Print and shaded views of the part. All mm, measured from the part's lowest x, y and z. A direction names the side the tool comes from. Round coordinates to 2 decimals unless told otherwise and drop trailing zeros. Loops run counter-clockwise (first coordinate to the right, second up) from the corner with the lowest first, then second, coordinate; pieces in that order, holes last. Notation, with made-up numbers: (-24.75, 26) - (-16.75, 26) arc R21 cw to (-16.75, 47) - close; hole circle Ø5 at (83.5, 71). An arc over 180 degrees is marked (long way). Use one line per item in the form item = value.
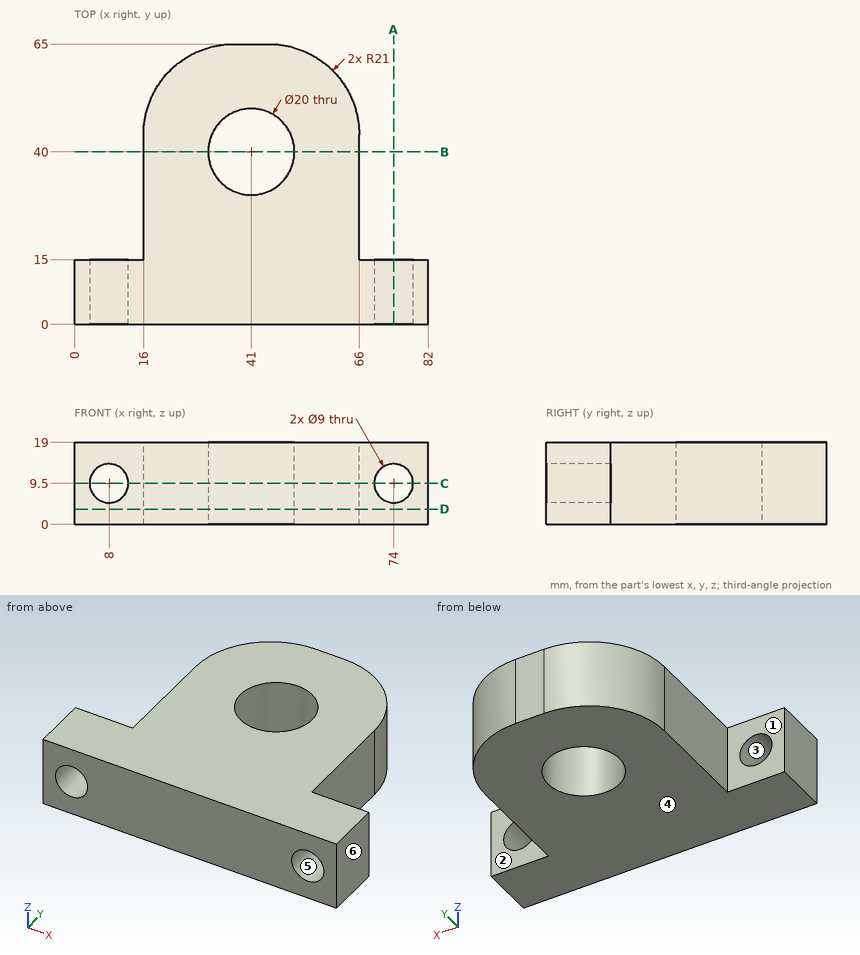
1) Flat gauge pins, fed straight in: pin 1 (1.5 mm diameter, centred on x = 10.5, z = 3.5, fed in from +Y); pin 2 (1 mm diameter, centred on y = 21, z = 7, fed in from +X); pin 3 (9.5 mm diameter, centred on y = 25, z = 10, fed in from -X). Where does each tip first touch, or does it go through?
Report:
pin_1 = 15
pin_2 = 66
pin_3 = 16
2) Slice it at C-C (z = 9.5). Write the cut outline in (x, y).
Report:
outline = (0, 0) - (3.5, 0) - (3.5, 15) - (0, 15) - close; (12.5, 0) - (69.5, 0) - (69.5, 15) - (66, 15) - (66, 44) arc R21 ccw to (45, 65) - (37, 65) arc R21 ccw to (16, 44) - (16, 15) - (12.5, 15) - close; (78.5, 0) - (82, 0) - (82, 15) - (78.5, 15) - close; hole circle Ø20 at (41, 40)
3) Tool access for the marked faces 1, 2 and 3: list every direction of +Z, -Z, +X, -X, +Y, -Y with a clear straight run to the whole face (end or side of a thin tool).
Report:
face_1 = +Z, -Z, -X, +Y
face_2 = +Z, -Z, +X, +Y
face_3 = +Y, -Y
4) Slice it at D-D (z = 3.5). Write the cut outline in (x, y).
Report:
outline = (0, 0) - (82, 0) - (82, 15) - (66, 15) - (66, 44) arc R21 ccw to (45, 65) - (37, 65) arc R21 ccw to (16, 44) - (16, 15) - (0, 15) - close; hole circle Ø20 at (41, 40)
5) Drill centre lines: probe 1 along Z at (x, y) = (74, 7); probe 2 along Y at (x, z) = (41, 7.5); probe 3 along Y at (x, z) = (71.5, 2.25). Where is each one in solid material? Low to high.
Report:
probe_1 = 0 to 5, 14 to 19
probe_2 = 0 to 30, 50 to 65
probe_3 = 0 to 15
6) Slice it at A-A (x = 74). Write the cut outline in (y, z).
Report:
outline = (0, 0) - (15, 0) - (15, 5) - (0, 5) - close; (0, 14) - (15, 14) - (15, 19) - (0, 19) - close
7) Two-plate mould, pull along Z, no slides. Class the marked faces 4, 5 and 6: +Z half, -Z half, draft (parallel to the pull), parting line (faces both ways), or undercut.
Report:
face_4 = -Z half
face_5 = undercut
face_6 = draft
8) Slice it at B-B (y = 40). Write the cut outline in (x, z).
Report:
outline = (16, 0) - (31, 0) - (31, 19) - (16, 19) - close; (51, 0) - (66, 0) - (66, 19) - (51, 19) - close
